from build123d import *

# Parameters (mm, degrees)
EXTRUDE_1_DEPTH = 10


with BuildPart() as part:
    # 草图1 → 凸台-拉伸1 (new body)
    with BuildSketch(Plane(origin=(0, 0, 0), x_dir=(1, 0, 0), z_dir=(0, 1, 0))):
        with BuildLine():
            ThreePointArc((156.5, 0), (152.985281374, 8.485281374), (144.5, 12))
            Line((144.5, 12), (144.5, 11.08))
            ThreePointArc((144.5, 11.08), (152.334743136, 7.834743136), (155.58, 0))
            ThreePointArc((155.58, 0), (152.334743136, -7.834743136), (144.5, -11.08))
            Line((144.5, -11.08), (144.5, -12))
            ThreePointArc((144.5, -12), (152.985281374, -8.485281374), (156.5, 0))
        make_face()
        with BuildLine():
            ThreePointArc((144.5, 12), (142.150531975, 11.767752547), (139.892006944, 11.08))
            Line((139.892006944, 11.08), (144.5, 11.08))
            Line((144.5, 11.08), (144.5, 12))
        make_face()
        with BuildLine():
            ThreePointArc((0, 12), (2.349468025, 11.767752547), (4.607993056, 11.08))
            Line((4.607993056, 11.08), (139.892006944, 11.08))
            ThreePointArc((139.892006944, 11.08), (142.150531975, 11.767752547), (144.5, 12))
            Line((144.5, 12), (0, 12))
        make_face()
        with BuildLine():
            Line((144.5, -11.08), (139.892006944, -11.08))
            ThreePointArc((139.892006944, -11.08), (142.150531975, -11.767752547), (144.5, -12))
            Line((144.5, -12), (144.5, -11.08))
        make_face()
        with BuildLine():
            Line((139.892006944, -11.08), (4.607993056, -11.08))
            ThreePointArc((4.607993056, -11.08), (2.349468025, -11.767752547), (0, -12))
            Line((0, -12), (144.5, -12))
            ThreePointArc((144.5, -12), (142.150531975, -11.767752547), (139.892006944, -11.08))
        make_face()
        with BuildLine():
            Line((0, 12), (0, 11.08))
            Line((0, 11.08), (4.607993056, 11.08))
            ThreePointArc((4.607993056, 11.08), (2.349468025, 11.767752547), (0, 12))
        make_face()
        with BuildLine():
            Line((4.607993056, -11.08), (0, -11.08))
            Line((0, -11.08), (0, -12))
            ThreePointArc((0, -12), (2.349468025, -11.767752547), (4.607993056, -11.08))
        make_face()
        with BuildLine():
            ThreePointArc((0, -11.08), (-11.08, 0), (0, 11.08))
            Line((0, 11.08), (0, 12))
            ThreePointArc((0, 12), (-12, 0), (0, -12))
            Line((0, -12), (0, -11.08))
        make_face()
    extrude(amount=EXTRUDE_1_DEPTH)


solid = part.part
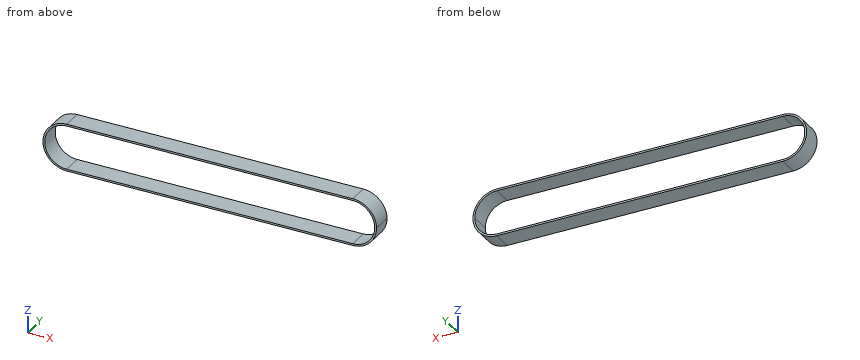
The model under review builds one solid part; all positions refer to its coordinate system, in mm. Give positions to 0.01 mm unless a question says otherwise; leave off trailing zeros. Loops run counter-clockwise (first coordinate to the right, second up) from the corner with the lowest first, then second, coordinate; pieces in that order, holes last. Notation, with made-up numbers: (-14.75, 31.25) -> (5.25, 31.25) arc R21 ccw to (5.25, 70.25) -> close; hole circle Ø2 at (46.25, -34.5). An arc over 180 degrees is marked (long way). Put each result on its own line as item: value. Start each with the question number.
1. Wall thickness on probe 1 along Z at (x, y) = (44, 3); probe 2 along X at (y, z) = (8, -1); probe 3 along X at (y, z) = (4.5, -2): over which ranges is each line inside the solid? List them lowest first.
2. We need section C-C on z = -2.75. State the section outline as (x, y) points, then the cut area to 3 significant figures.
3. We need section B-B on x = 88. State the section outline as (y, z) points, then the cut area to 3 significant figures.
4. Clearance check with flat-ended pins moving along their axes: P1, Ø1, axis at y = 2, z = 7, coming from the +X side; P2, Ø1, axis at y = 1, z = -7.5, coming from the +X side. State where each tip first meets the part, or that it passes through.
5. We need section A-A on y = 8.25. State the section outline as (x, z) points.
Determined:
1. probe 1: -12 to -11.08, 11.08 to 12
1. probe 2: -11.96 to -11.03, 155.53 to 156.46
1. probe 3: -11.83 to -10.9, 155.4 to 156.33
2. outline: (-11.68, 0) -> (-10.73, 0) -> (-10.73, 10) -> (-11.68, 10) -> close; (155.23, 0) -> (156.18, 0) -> (156.18, 10) -> (155.23, 10) -> close
2. area: 18.9 mm^2
3. outline: (0, -12) -> (10, -12) -> (10, -11.08) -> (0, -11.08) -> close; (0, 11.08) -> (10, 11.08) -> (10, 12) -> (0, 12) -> close
3. area: 18.4 mm^2
4. P1: x = 154.59
4. P2: x = 154.25
5. outline: (0, -12) -> (144.5, -12) arc R12 ccw to (144.5, 12) -> (0, 12) arc R12 ccw to start; hole (0, -11.08) -> (144.5, -11.08) arc R11.08 ccw to (144.5, 11.08) -> (0, 11.08) arc R11.08 ccw to start
